Can you work these out from the model? Positions are in its coordinate system, mm. A direction names the side the tool comes from. Coordinates: 2 decimals unless noted, no trailing zeros. Write each loop counter-clockwise with the first axis right and the second up, starting at its lowest first coordinate (ties: lowest second). Pieces come first, ordered by that corner, then holes. Notation, with made-up numbers: M 58,2.25 L 66,2.25 A35 cw 66,37.25 Z; hole C -17.75,88.5 d5. An arc over 180 degrees is marked long. Answer as a JSON object with one key per item and string values. Group by question number.
from build123d import *
from OCP.BRepFilletAPI import BRepFilletAPI_MakeChamfer

# Parameters (mm, degrees)
SKETCH1_R           = 7.774999999999999
SKETCH1_R_2         = 1.6319499986664014
BOSS_EXTRUDE1_DEPTH = 3
SKETCH1_3_R         = 1.6319499986664014
SKETCH1_3_R_2       = 7.774999999999999
BOSS_EXTRUDE2_DEPTH = 1.6
CHAMFER1_SIZE       = 2
CHAMFER1_SIZE2      = 1.5
CHAMFER2_SIZE2      = 1.4
CHAMFER2_SIZE       = 9
CHAMFER3_SIZE       = 1.4
CHAMFER3_SIZE_2     = 9


# Some blends are built 0.0001 mm under size
with BuildPart() as part:
    # Sketch1 → Boss-Extrude1 (new body)
    with BuildSketch(Plane.XY):
        with BuildLine():
            Line((-15.995731683346964, -4.286043386897756), (-19.531020207564957, -5.233321091972986))
            ThreePointArc((-19.53102020756496, -5.233321091972988), (-18.780139119855487, -7.49364895353884), (-17.76867749721403, -9.650000000000002))
            Line((-17.76867749721403, -9.65), (13.457752412643053, -9.650000000000004))
            ThreePointArc((13.457752412643053, -9.650000000000004), (16.29203049556925, -2.967042691206455), (15.995731683346978, 4.286043386897719))
            Line((15.995731683346953, 4.286043386897752), (19.531020207564957, 5.233321091972986))
            ThreePointArc((19.531020207564957, 5.233321091972985), (18.78013911985548, 7.493648953538841), (17.768677497214025, 9.650000000000002))
            Line((17.76867749721402, 9.650000000000002), (-13.457752412643053, 9.650000000000002))
            ThreePointArc((-13.457752412643051, 9.650000000000002), (-16.292030495569243, 2.967042691206453), (-15.995731683346973, -4.286043386897722))
        make_face()
        Circle(SKETCH1_R, mode=Mode.SUBTRACT)
        with Locations((11.610000000000001, 2.84e-15)):
            Circle(SKETCH1_R_2, mode=Mode.SUBTRACT)
        with Locations((-11.609999999999998, 0)):
            Circle(SKETCH1_R_2, mode=Mode.SUBTRACT)
    extrude(amount=BOSS_EXTRUDE1_DEPTH)

    # Sketch1<3> → Boss-Extrude2 (add)
    with BuildSketch(Plane.XY):
        with BuildLine():
            Line((-17.768677497214025, -9.649999999999999), (17.76867749721402, -9.650000000000002))
            ThreePointArc((17.76867749721402, -9.650000000000002), (20.22, 0), (17.76867749721402, 9.650000000000002))
            Line((17.76867749721402, 9.650000000000002), (-17.768677497214025, 9.649999999999999))
            ThreePointArc((-17.768677497214025, 9.649999999999999), (-20.220000000000002, 2.48e-15), (-17.768677497214025, -9.649999999999999))
        make_face()
        with Locations((-11.609999999999998, 0)):
            Circle(SKETCH1_3_R, mode=Mode.SUBTRACT)
        with Locations((11.610000000000001, 2.84e-15)):
            Circle(SKETCH1_3_R, mode=Mode.SUBTRACT)
        Circle(SKETCH1_3_R_2, mode=Mode.SUBTRACT)
    extrude(amount=BOSS_EXTRUDE2_DEPTH)

    # Chamfer1: one chamfer whose edges measure the first distance from different faces: ONE call of the kernel's chamfer builder (chamfer() names one face for all edges)
    chamfer1_edges_1 = [part.edges().sort_by_distance(p)[0] for p in [
        (-13.2419499986664, 2e-16, 0),
    ]]
    chamfer1_side_1 = [part.faces().sort_by_distance(p)[0] for p in [
        (-13.2419499986664, 2e-16, 1.5),
    ]]
    chamfer1_edges_2 = [part.edges().sort_by_distance(p)[0] for p in [
        (9.9780500013336, 3.04e-15, 0),
    ]]
    chamfer1_side_2 = [part.faces().sort_by_distance(p)[0] for p in [
        (9.9780500013336, 3.04e-15, 1.5),
    ]]
    chamfer1 = BRepFilletAPI_MakeChamfer(part.part.solid().wrapped)
    for e in chamfer1_edges_1:
        chamfer1.Add(CHAMFER1_SIZE, CHAMFER1_SIZE2, e.wrapped, chamfer1_side_1[0].wrapped)  # the first distance lies on this face
    for e in chamfer1_edges_2:
        chamfer1.Add(CHAMFER1_SIZE, CHAMFER1_SIZE2, e.wrapped, chamfer1_side_2[0].wrapped)  # the first distance lies on this face
    add(Compound.cast(chamfer1.Shape()), mode=Mode.REPLACE)

    # Chamfer2
    chamfer2_edges = [part.edges().sort_by_distance(p)[0] for p in [
        (-17.763375945455962, -4.759682239435371, 1.6),
    ]]
    chamfer2_side = [part.faces().sort_by_distance(p)[0] for p in [
        (-17.770622878718832, -4.732636316299277, 1.6),
    ]]
    chamfer(chamfer2_edges, length=CHAMFER2_SIZE - 0.0001, length2=CHAMFER2_SIZE2 - 0.0001, reference=chamfer2_side[0])  # a hair under: the kernel refuses the full size

    # Chamfer3
    # the kernel refuses this chamfer: 9, 1.4 mm, written as the material it adds along each edge
    with BuildSketch(Plane(origin=(-6.596997055985572, -1.7676600336218398, 1.6), x_dir=(-0.06145306059893889, 0.22934594443584813, 0.9714030878651004), z_dir=(0.9659258262890681, 0.2588190451025218, 0))) as chamfer3_piece_1_section:
        Polygon((CHAMFER3_SIZE * 0.971403087865, CHAMFER3_SIZE * 0.237436393348), (-CHAMFER3_SIZE_2 * 0.237436393348, CHAMFER3_SIZE_2 * 0.971403087865), (0, 0), align=None)
    chamfer3_piece_1 = extrude(amount=50.43942782859462, mode=Mode.PRIVATE)
    chamfer3_piece_1 = split(chamfer3_piece_1, bisect_by=Plane(origin=(18.152512128886663, 1.3968714371036275, 3), z_dir=(0, 0, -1)), keep=Keep.TOP, mode=Mode.PRIVATE)
    chamfer3_piece_1 = chamfer3_piece_1 & Plane(origin=(-9.0949e-13, -3.5172e-13, 1.9557710563894077), x_dir=(0.9659258262890668, 0.2588190451025265, 0), z_dir=(0, 0, -1)) * Cylinder(20.22000000000097, 136, mode=Mode.PRIVATE)
    chamfer3_piece_1 = chamfer3_piece_1 - Plane(origin=(2.665e-14, -4.11e-15, 1.9557710563894077), x_dir=(0.8126662084929376, -0.5827294685990347, 0), z_dir=(0, 0, -1)) * Cylinder(16.559999999999974, 136, mode=Mode.PRIVATE)
    add(chamfer3_piece_1)


solid = part.part
Q1. If we section it at D-D on x = -11.61: List the corners of the cut face in (y, z) for me.
Q2. Please list where these lines run through material, in increasing order: L1, parallel to Y at x = 0, z = 1.5 (3 decimals); L2, parallel to Y at x = 11.61, z = 2.3; L3, parallel to Z at x = 17.5, y = -4.75.
Q3. If we section it at C-C on z = 2.4: Give the number of separate pieces and of enclosed holes in the cut face, and give its area (3 significant figures).
Q4. Will these pins go through, and if not, where does the flat tip stop? pin 1 (1.5 mm diameter, centred on y = 4, z = 1.5, fed in from +X); pin 2 (5 mm diameter, centred on x = 11.61, y = 0, fed in from -Z); pin 3 (1 mm diameter, centred on y = 0.5, z = 2, fed in from +X); pin 4 (10 mm diameter, centred on x = 0.5, y = 2.5, fed in from +Z).
Q5. We'd pull the mould along Y, two halves only. Please class faces 6 (the cylindrical face through (-1.69, -7.59, 1.48)), 7 (the flat face through (0, 9.65, 1)), 8 (the cylindrical face through (20.08, 2.37, 1.15)), 9 (the flat face through (-5, 7, 3)): pulls with the +Y half, pulls with the -Y half, needs draft (parallel to the pull), parting line crosses it, or undercut.
Q6. If we section it at A-A on x = 0: List the corners of the cut face in (y, z) for me (3 decimals), and give its area (4 significant figures).
Q7. If we section it at B-B on y = -7: List the corners of the cut face in (x, z) for me, and give its area (3 significant figures).
Q8. On a 3-axis mill with a long thin cutter (end or side, diameter ignored), from which of +Z, -Z, +X, -X, +Y, -Y can I reach the whole of each face in a straight line? I mean faces 1 (the flat face through (-17, 7, 1.6)), 2 (the cylindrical face through (-15.894, 4.649, 2.446)), 3 (the conical face through (-10.814, -1.531, 1.875)), 4 (the cylindrical face through (15.894, -4.649, 2.446)), 5 (the flat face through (17, -7, 1.6)). Say none if no direction works.
Reply:
{
 "1": {"outline": "M -9.65,0 L -3.13,0 L -1.63,2 L -1.63,3 L -9.65,3 Z; M 1.63,2 L 3.13,0 L 9.65,0 L 9.65,3 L 1.63,3 Z"},
 "2": {"L1": "-9.65 to -7.775, 7.775 to 9.65", "L2": "-9.65 to -1.63, 1.63 to 9.65", "L3": "0 to 1.6"},
 "3": {"separate pieces": "1", "enclosed holes": "3", "area": "462 mm^2"},
 "4": {"pin 1": "x = 19.96", "pin 2": "z = 0.84", "pin 3": "x = 20.22", "pin 4": "through"},
 "5": {"face 6": "undercut", "face 7": "pulls with the +Y half", "face 8": "parting line crosses it", "face 9": "needs draft"},
 "6": {"outline": "M -9.65,0 L -7.775,0 L -7.775,3 L -9.65,3 Z; M 7.775,0 L 9.65,0 L 9.65,3 L 7.775,3 Z", "area": "11.25 mm^2"},
 "7": {"outline": "M -18.97,0 L -3.38,0 L -3.38,3 L -18.97,3 Z; M 3.38,0 L 18.97,0 L 18.97,1.6 L 15.01,1.6 L 15.01,3 L 3.38,3 Z", "area": "88.0 mm^2"},
 "8": {"face 1": "+Z, -X, +Y", "face 2": "+Z, -X", "face 3": "-Z", "face 4": "+Z, +X", "face 5": "+Z, +X, -Y"}
}
